Geometry check sheet. Reference: the model listing, model coordinates, mm. A direction names the side the tool comes from. Round coordinates to 2 decimals unless told otherwise and drop trailing zeros. Loops run counter-clockwise (first coordinate to the right, second up) from the corner with the lowest first, then second, coordinate; pieces in that order, holes last. Notation, with made-up numbers: M 5,38.5 L 54,38.5 A14 ccw 54,53.5 Z; hole C -5.75,-39.75 d8. An arc over 180 degrees is marked long. Use one line per item in the form item = value. Start each with the question number.
1. Cross-section at D-D (x = 9.75). Record the boundary of the cut face in (y, z) (3 decimals), then the cut area to 3 significant figures.
2. Material ranges on line 1 (Z direction, x = 6.35, y = -1.55); line 2 (X direction, y = -1.9, z = 0); line 3 (Z direction, x = 5.5, y = -0.55), recorded low to high.
3. Set-up check for faces 4 (the flat face through (12.7, -2, 25)), 5 (the flat face through (-1, -2, -21.368)), 6 (the flat face through (0, -2, -31)), 7 (the flat face through (0, -2, 16)): record each of +Z, -Z, +X, -X, +Y, -Y from which the full face is reachable in a straight line by a thin tool's end or side.
4. Draft check along X on faces 1 (the flat face through (-0.783, -1.565, -23.89)), 2 (the cylindrical face through (4.759, -1.565, 42.734)), 3 (the flat face through (4.762, -2, -23)). Enter one of: pulls with the +X half, pulls with the -X half, needs draft (parallel to the pull), parting line crosses it, or undercut.
5. Cross-section at C-C (z = -16). Record the boundary of the cut face in (x, y) (1 decimal), then the cut area to 3 significant figures.
6. Cross-section at A-A (y = -2.1). State how many separate pieces and enclosed holes the cut face has, then the cut area to 3 significant figures.
7. Go/stop test with flat-tipped pins: pin 1 (1 mm diameter, centred on x = 3, z = 31, fed in from +Y); pin 2 (1.3 mm diameter, centred on x = -1, y = -2, fed in from -Z); pin 3 (0.6 mm diameter, centred on y = -1.5, z = -26, fed in from -X). Record where each tip stops, or that it passes through.
8. Cross-section at B-B (x = 6.35). Record the boundary of the cut face in (y, z) (3 decimals), then the cut area to 3 significant figures.
```python
from build123d import *

# Parameters (mm, degrees)
F0_R     = 2.159
F1_DEPTH = 3.175


with BuildPart() as f1:
    # F0 (on Front) → F1 (new body)
    with BuildSketch(Plane.XZ):
        with BuildLine():
            ThreePointArc((4.191, 0), (6.35, 2.159), (8.509, 0))
            Line((8.509, 0), (12.7, 0))
            Line((12.7, 0), (12.7, 50.8))
            Line((12.7, 50.8), (0, 50.8))
            Line((0, 50.8), (0, 0))
            Line((0, 0), (4.191, 0))
        make_face()
        with Locations((6.35, 41.275)):
            Circle(F0_R, mode=Mode.SUBTRACT)
        with BuildLine():
            Line((12.7, 0), (8.509, 0))
            ThreePointArc((8.509, 0), (6.35, -2.159), (4.191, 0))
            Line((4.191, 0), (0, 0))
            Line((0, 0), (0, -18.828153))
            Line((0, -18.828153), (0, -21.368153))
            Line((0, -21.368153), (0, -22.638153))
            Line((0, -22.638153), (0, -25.178153))
            Line((0, -25.178153), (0, -26.448153))
            Line((0, -26.448153), (0, -28.988153))
            Line((0, -28.988153), (0, -32.798153))
            Line((0, -32.798153), (4.7625, -32.798153))
            Line((4.7625, -32.798153), (4.7625, -13.748153))
            Line((4.7625, -13.748153), (12.7, 0))
        make_face()
        with BuildLine():
            Line((0, 50.8), (12.7, 50.8))
            ThreePointArc((12.7, 50.8), (6.35, 57.15), (0, 50.8))
        make_face()
        Polygon((0, -21.368153), (0, -18.828153), (-1.5875, -21.368153), align=None)
        Polygon((-1.5875, -28.988153), (0, -28.988153), (0, -26.448153), align=None)
        Polygon((0, -25.178153), (0, -22.638153), (-1.5875, -25.178153), align=None)
    extrude(amount=F1_DEPTH)


solid = f1.part
```
Reported:
q1.outline = M -3.175,-5.11 L 0,-5.11 L 0,56.163 L -3.175,56.163 Z
q1.area = 195 mm²
q2.line_1 = -11 to -2.16, 2.16 to 39.12, 43.43 to 57.15
q2.line_2 = 0 to 4.19, 8.51 to 12.7
q2.line_3 = -12.47 to -1.98, 1.98 to 39.29, 43.26 to 57.09
q3.face_4 = +Z, -Z, +X, +Y, -Y
q3.face_5 = -X, +Y, -Y
q3.face_6 = -Z, -X, +Y, -Y
q3.face_7 = +Z, -X, +Y, -Y
q4.face_1 = pulls with the -X half
q4.face_2 = undercut
q4.face_3 = pulls with the +X half
q5.outline = M 0,-3.2 L 4.8,-3.2 L 4.8,0 L 0,0 Z
q5.area = 15.1 mm²
q6.separate_pieces = 1
q6.enclosed_holes = 2
q6.area = 896 mm²
q7.pin_1 = 0
q7.pin_2 = -28.99
q7.pin_3 = 0
q8.outline = M -3.175,-10.999 L 0,-10.999 L 0,-2.159 L -3.175,-2.159 Z; M -3.175,2.159 L 0,2.159 L 0,39.116 L -3.175,39.116 Z; M -3.175,43.434 L 0,43.434 L 0,57.15 L -3.175,57.15 Z
q8.area = 189 mm²
